Autodesk Inventor part; units mm, degrees
ref_plane "YZ Plane" through (0, 0, 0) normal (1, 0, 0) x (0, 1, 0)
ref_plane "XZ Plane" through (0, 0, 0) normal (0, 1, 0) x (-1, 0, 0)
ref_plane "XY Plane" through (0, 0, 0) normal (0, 0, 1) x (1, 0, 0)
sketch "Sketch1" plane through (0, 0, 0) normal (0, 1, 0) x (-1, 0, 0)
  line L0 (-20, 22) -> (-22, 20)
  line L1 (-20, -22) -> (20, -22)
  line L2 (-35, 51.3397) -> (-35, -51.3397)
  arc A0 (35, 51.3397) -> (21.3397, 65) centre (30, 60) ccw
  arc A1 (21.3397, -65) -> (35, -51.3397) centre (30, -60) ccw
  line L3 (22, 20) -> (20, 22)
  line L4 (-22, 20) -> (-22, -20)
  line L5 (20, -22) -> (22, -20)
  arc A2 (-21.3397, 65) -> (-35, 51.3397) centre (-30, 60) ccw
  line L6 (35, -51.3397) -> (35, 51.3397)
  line L7 (20, 22) -> (-20, 22)
  line L8 (-22, -20) -> (-20, -22)
  arc A3 (-35, -51.3397) -> (-21.3397, -65) centre (-30, -60) ccw
  line L9 (21.3397, 65) -> (-21.3397, 65)
  line L10 (-21.3397, -65) -> (21.3397, -65)
  line L11 (22, -20) -> (22, 20)
extrude "Extrusion1" add sketch "Sketch1" against normal blind 4.064
hole "Hole22" at (0, -4.064, 57.5) direction (0, 1, 0) diameter 4.5 depth 4.064
hole "Hole21" at (0, -4.064, -57.5) direction (0, 1, 0) diameter 4.5 depth 4.064
hole "Hole20" at (-16, 0, -46) direction (0, -1, 0) diameter 4.5 depth 4.064
hole "Hole19" at (-16, 0, -30) direction (0, -1, 0) diameter 4.5 depth 4.064
hole "Hole18" at (16, 0, -46) direction (0, -1, 0) diameter 4.5 depth 4.064
hole "Hole17" at (16, 0, -30) direction (0, -1, 0) diameter 4.5 depth 4.064
hole "Hole16" at (16, 0, 30) direction (0, -1, 0) diameter 4.5 depth 4.064
hole "Hole15" at (16, 0, 46) direction (0, -1, 0) diameter 4.5 depth 4.064
hole "Hole14" at (-16, 0, 30) direction (0, -1, 0) diameter 4.5 depth 4.064
hole "Hole13" at (-16, 0, 46) direction (0, -1, 0) diameter 4.5 depth 4.064
hole "Hole12" at (27.5, 0, -15) direction (0, -1, 0) diameter 4.5 depth 4.064
sketch "Sketch12" plane through (0, 0, 0) normal (0, 1, 0) x (-1, 0, 0)
  point P0 (-27.5, -15)
hole "Hole11" at (27.5, 0, 15) direction (0, -1, 0) diameter 4.5 depth 4.064
sketch "Sketch11" plane through (0, 0, 0) normal (0, 1, 0) x (-1, 0, 0)
  point P0 (16, 46)
hole "Hole10" at (-27.5, 0, -15) direction (0, -1, 0) diameter 4.5 depth 4.064
sketch "Sketch10" plane through (0, 0, 0) normal (0, 1, 0) x (-1, 0, 0)
  point P0 (16, 30)
hole "Hole9" at (-24.3431, 0, -54.3431) direction (0, -1, 0) diameter 4.5 depth 4.064
sketch "Sketch9" plane through (0, 0, 0) normal (0, 1, 0) x (-1, 0, 0)
  point P0 (-16, 46)
hole "Hole8" at (24.3431, 0, -54.3431) direction (0, -1, 0) diameter 4.5 depth 4.064
sketch "Sketch8" plane through (0, 0, 0) normal (0, 1, 0) x (-1, 0, 0)
  point P0 (-16, 30)
hole "Hole7" at (24.3431, 0, 54.3431) direction (0, -1, 0) diameter 4.5 depth 4.064
sketch "Sketch7" plane through (0, 0, 0) normal (0, 1, 0) x (-1, 0, 0)
  point P0 (-16, -30)
hole "Hole6" at (-24.3431, 0, 54.3431) direction (0, -1, 0) diameter 4.5 depth 4.064
sketch "Sketch6" plane through (0, 0, 0) normal (0, 1, 0) x (-1, 0, 0)
  point P0 (-16, -46)
hole "Hole5" at (-30, -4.064, 60) direction (0, 1, 0) diameter 4.5 depth 4.064
sketch "Sketch5" plane through (0, 0, 0) normal (0, 1, 0) x (-1, 0, 0)
  point P0 (16, -30)
hole "Hole4" at (30, -4.064, 60) direction (0, 1, 0) diameter 4.5 depth 4.064
sketch "Sketch4" plane through (0, 0, 0) normal (0, 1, 0) x (-1, 0, 0)
  point P0 (16, -46)
hole "Hole3" at (30, -4.064, -60) direction (0, 1, 0) diameter 4.5 depth 4.064
sketch "Sketch3" plane through (0, -4.064, 0) normal (0, -1, 0) x (1, 0, 0)
  point P0 (0, -57.5)
hole "Hole2" at (-30, -4.064, -60) direction (0, 1, 0) diameter 4.5 depth 4.064
sketch "Sketch2" plane through (0, -4.064, 0) normal (0, -1, 0) x (1, 0, 0)
  point P0 (0, 57.5)
hole "Hole1" at (-27.5, 0, 15) direction (0, -1, 0) diameter 4.5 depth 4.064
sketch "Sketch13" plane through (0, 0, 0) normal (0, 1, 0) x (-1, 0, 0)
  point P0 (-27.5, 15)
sketch "Sketch14" plane through (0, 0, 0) normal (0, 1, 0) x (-1, 0, 0)
  point P0 (27.5, -15)
sketch "Sketch15" plane through (0, 0, 0) normal (0, 1, 0) x (-1, 0, 0)
  point P0 (24.3431, -54.3431)
sketch "Sketch16" plane through (0, 0, 0) normal (0, 1, 0) x (-1, 0, 0)
  point P0 (-24.3431, -54.3431)
sketch "Sketch17" plane through (0, 0, 0) normal (0, 1, 0) x (-1, 0, 0)
  point P0 (-24.3431, 54.3431)
sketch "Sketch18" plane through (0, 0, 0) normal (0, 1, 0) x (-1, 0, 0)
  point P0 (24.3431, 54.3431)
sketch "Sketch19" plane through (0, -4.064, 0) normal (0, -1, 0) x (1, 0, 0)
  point P0 (-30, 60)
sketch "Sketch20" plane through (0, -4.064, 0) normal (0, -1, 0) x (1, 0, 0)
  point P0 (30, 60)
sketch "Sketch21" plane through (0, -4.064, 0) normal (0, -1, 0) x (1, 0, 0)
  point P0 (30, -60)
sketch "Sketch22" plane through (0, -4.064, 0) normal (0, -1, 0) x (1, 0, 0)
  point P0 (-30, -60)
sketch "Sketch23" plane through (0, 0, 0) normal (0, 1, 0) x (-1, 0, 0)
  point P0 (27.5, 15)
properties part number "Piston Feed frame" material "Aluminum 6061"
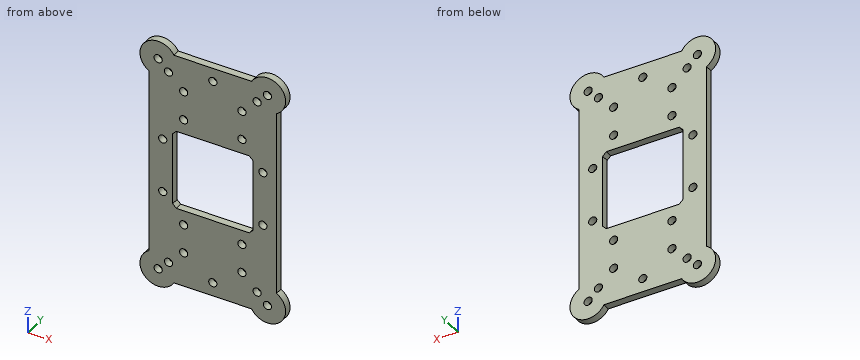
For this review, take the finished solid that the model builds, in its own axes (mm). Round coordinates to 2 decimals unless told otherwise and drop trailing zeros. Write each loop counter-clockwise with the first axis right and the second up, starting at its lowest first coordinate (ties: lowest second). Pieces come first, ordered by that corner, then holes. Notation, with made-up numbers: (69.25, 48.5) - (105.25, 48.5) arc R16 ccw to (105.25, 74.5) - close; hole circle Ø11 at (-31.75, 40). An arc over 180 degrees is marked (long way). Use CSV: the item, a comma, the result in double quotes.
1) Add section C-C on x = -5. Write out the cut boundary in (y, z), and give its area (3 significant figures).
Conclusion:
outline,"(-4.06, -65) - (0, -65) - (0, -22) - (-4.06, -22) - close; (-4.06, 22) - (0, 22) - (0, 65) - (-4.06, 65) - close"
area,"350 mm^2"
2) Add section A-A on x = 16. Write out the cut boundary in (y, z), and give its area (3 significant figures).
Conclusion:
outline,"(-4.06, -65) - (0, -65) - (0, -48.25) - (-4.06, -48.25) - close; (-4.06, -43.75) - (0, -43.75) - (0, -32.25) - (-4.06, -32.25) - close; (-4.06, -27.75) - (0, -27.75) - (0, -22) - (-4.06, -22) - close; (-4.06, 22) - (0, 22) - (0, 27.75) - (-4.06, 27.75) - close; (-4.06, 32.25) - (0, 32.25) - (0, 43.75) - (-4.06, 43.75) - close; (-4.06, 48.25) - (0, 48.25) - (0, 65) - (-4.06, 65) - close"
area,"276 mm^2"
3) Add section B-B on z = 15. Write out the cut boundary in (x, y), and give its area (3 significant figures).
Conclusion:
outline,"(-35, -4.06) - (-29.75, -4.06) - (-29.75, 0) - (-35, 0) - close; (-25.25, -4.06) - (-22, -4.06) - (-22, 0) - (-25.25, 0) - close; (22, -4.06) - (25.25, -4.06) - (25.25, 0) - (22, 0) - close; (29.75, -4.06) - (35, -4.06) - (35, 0) - (29.75, 0) - close"
area,"69.1 mm^2"
4) Clearance check with flat-ended pins moving along their axes: pin 1 Ø4 at (x, z) = (27.5, 15) entering from +Y; pin 2 Ø5 at (x, z) = (16, -30) entering from -Y; pin 3 Ø2 at (y, z) = (-1, 3.5) entering from +X; pin 4 Ø1.2 at (x, y) = (7, -1.5) entering from +Z. State where each tip first meets the part, or that it passes through.
Conclusion:
pin 1,"passes through"
pin 2,"stops at y = -4.06"
pin 3,"stops at x = 35"
pin 4,"stops at z = 65"
5) Wall thickness on line 1 along Z through (x, y) = (30, -1.75); line 2 along X through (y, z) = (-3.25, 2); line 3 along X through (y, z) = (-1.75, 15): over which ranges is each line inside the solid? List them lowest first. Write a range as from..to.
Conclusion:
line 1,"z = -70..-62.25, -57.75..57.75, 62.25..70"
line 2,"x = -35..-22, 22..35"
line 3,"x = -35..-29.75, -25.25..-22, 22..25.25, 29.75..35"
6) Add section D-D on z = 30. Write out the cut boundary in (x, y), and give its area (3 significant figures).
Conclusion:
outline,"(-35, -4.06) - (-18.25, -4.06) - (-18.25, 0) - (-35, 0) - close; (-13.75, -4.06) - (13.75, -4.06) - (13.75, 0) - (-13.75, 0) - close; (18.25, -4.06) - (35, -4.06) - (35, 0) - (18.25, 0) - close"
area,"248 mm^2"
